from build123d import *

# Parameters (mm, degrees)
EXTRUSION1_DEPTH = 38.1


with BuildPart() as part:
    # Sketch1 → Extrusion1 (new body)
    with BuildSketch(Plane.XY):
        with BuildLine():
            Line((2.416962135, 2.058863531), (3.1501433, 3.32877056))
            Line((3.1501433, 3.32877056), (1.336888207, 4.375653876))
            Line((1.336888207, 4.375653876), (0.609587103, 3.115931412))
            ThreePointArc((0.609587103, 3.115931412), (-1.572031269, 2.758503705), (-2.991509188, 1.063718843))
            Line((-2.991509188, 1.063718843), (-4.457871519, 1.063718843))
            Line((-4.457871519, 1.063718843), (-4.457871519, -1.030047788))
            Line((-4.457871519, -1.030047788), (-3.003269311, -1.030047788))
            ThreePointArc((-3.003269311, -1.030047788), (-1.60291865, -2.740670867), (0.574547053, -3.122582374))
            Line((0.574547053, -3.122582374), (1.307728219, -4.392489404))
            Line((1.307728219, -4.392489404), (3.120983311, -3.345606088))
            Line((3.120983311, -3.345606088), (2.393682207, -2.085883623))
            ThreePointArc((2.393682207, -2.085883623), (3.174949919, -0.017832838), (2.416962135, 2.058863531))
        make_face()
    extrude(amount=EXTRUSION1_DEPTH)


solid = part.part
Build history of the part. All positions in model axes, mm. A direction names the side the tool comes from. Give positions to 0.01 mm unless a question says otherwise; leave off trailing zeros. Loops run counter-clockwise (first coordinate to the right, second up) from the corner with the lowest first, then second, coordinate; pieces in that order, holes last. Notation, with made-up numbers: (-35, 53.5) -> (-23, 53.5) arc R8 ccw to (-23, 65.5) -> close; hole circle Ø8 at (2, 44.5). An arc over 180 degrees is marked (long way). Answer in a Markdown table with one row per item.
Item 1: Tool access for faces 1 (the flat face through (-4, 1.064, 19)), 2 (the flat face through (0, 0, 38.1)), 3 (the flat face through (-4, -1.03, 19)), 4 (the flat face through (2.202, -3.876, 18.783)), 5 (the flat face through (2.778, 2.685, 18.783)): list every direction of +Z, -Z, +X, -X, +Y, -Y with a clear straight run to the whole face (end or side of a thin tool).
Findings below:
| item | result |
|---|---|
| face 1 | +Z, -Z, -X, +Y |
| face 2 | +Z, +X, -X, +Y, -Y |
| face 3 | +Z, -Z, -X, -Y |
| face 4 | +Z, -Z, +X, -Y |
| face 5 | +Z, -Z, +X |
Item 2: Slice it at B-B on x = -0.5. Write the cut outline in (y, z).
Findings below:
| item | result |
|---|---|
| outline | (-3.14, 0) -> (3.14, 0) -> (3.14, 38.1) -> (-3.14, 38.1) -> close |
Item 3: Mould opens along Y. For faces 6 (the cylindrical face through (-1.63, -2.725, 18.783)), 7 (the flat face through (0.978, 3.755, 18.783)), 8 (the flat face through (2.76, -2.72, 18.78)) say: pulls with the +Y half, pulls with the -Y half, needs draft (parallel to the pull), parting line crosses it, or undercut.
Findings below:
| item | result |
|---|---|
| face 6 | pulls with the -Y half |
| face 7 | pulls with the +Y half |
| face 8 | undercut |
Item 4: Flat gauge pins, fed straight in: P1, Ø1.2, axis at x = -3.5, z = 22, coming from the -Y side; P2, Ø1.6, axis at x = -3.5, z = 23.5, coming from the +Y side; P3, Ø1.5, axis at x = -3, z = 15, coming from the +Y side. Where does each tip first touch, or does it go through?
Findings below:
| item | result |
|---|---|
| P1 | stops at y = -1.29 |
| P2 | stops at y = 1.67 |
| P3 | stops at y = 2.24 |
Item 5: Probe line 1 along Y through (x, z) = (0, 30) (3 decimals); line 2 along X through (y, z) = (2, 20); line 3 along Y through (x, z) = (-2.5, 7.5). List the from-to ranges inside material, lowest first. Write a range as [from, to].
Findings below:
| item | result |
|---|---|
| line 1 | y = [-3.175, 3.175] |
| line 2 | x = [-2.47, 2.47] |
| line 3 | y = [-1.96, 1.96] |
Item 6: Slice it at C-C on y = -2.5. Write the cut outline in (x, z), plus the area to 3 significant figures.
Findings below:
| item | result |
|---|---|
| outline | (-1.96, 0) -> (2.63, 0) -> (2.63, 38.1) -> (-1.96, 38.1) -> close |
| area | 175 mm² |
